Here's how the part is built. I have some questions about the finished solid (model axes, mm). A direction names the side the tool comes from. Coordinates: 2 decimals unless noted, no trailing zeros. Loops run counter-clockwise (first coordinate to the right, second up) from the corner with the lowest first, then second, coordinate; pieces in that order, holes last. Notation, with made-up numbers: (51.5, 4) - (76.5, 4) arc R13 ccw to (76.5, 20) - close; hole circle Ø8 at (-17, -17.75). An arc over 180 degrees is marked (long way). Use a Markdown table: item, result.
```python
from build123d import *
from build123d import SkipClean  # not in build123d's __all__

# Parameters (mm, degrees)
F0_R     = 10.7
F1_DEPTH = 30
F2_R     = 6
F4_DEPTH = 10.701
F5_DEPTH = 10.7010001
F6_W     = 6.2500013784
F6_H     = 36.9480545221
F6_W_2   = 6.8020046502
F6_H_2   = 40.0000055429
F7_DEPTH = 24
F8_R     = 2


# Not quite as in the source:
# - after a boolean that leaves OpenCascade's solid faulty, fix() repairs it


with BuildPart() as f1:
    # F0 (on Top) → F1 (new body)
    with BuildSketch(Plane.XY):
        Circle(F0_R)
    extrude(amount=-F1_DEPTH)

    # F2
    f2_edges = [f1.edges().sort_by_distance(p)[0] for p in [
        (-10.7, 0, -30),
    ]]
    fillet(f2_edges, radius=F2_R)

    # F3 (on Right) → F4 (cut, through all)
    with BuildSketch(Plane.YZ):
        with BuildLine():
            ThreePointArc((0, -12.2), (-3.3941125497, -20.3941125497), (4.8, -17))
            ThreePointArc((4.8, -17), (3.3941125497, -13.6058874503), (0, -12.2))
        make_face()
    extrude(amount=-F4_DEPTH, mode=Mode.SUBTRACT)

    # F5 (cut, through all): a face of the model
    f5_faces = [f1.faces().sort_by_distance(p)[0] for p in [
        (0, 0, -17),
    ]]
    with SkipClean():  # cleaning this boolean's faces spoils the solid; the shape is the same uncleaned
        extrude(f5_faces, amount=-F5_DEPTH, mode=Mode.SUBTRACT)

    # F6 (on face) → F7 (cut)
    with BuildSketch(Plane(origin=(0, 0, -30), x_dir=(1, 0, 0), z_dir=(0, 0, -1))):
        with Locations((-8.1250006892, 1.5259755104)):
            Rectangle(F6_W, F6_H)
        with Locations((8.4010023251, 0)):
            Rectangle(F6_W_2, F6_H_2)
    extrude(amount=-F7_DEPTH, mode=Mode.SUBTRACT)

    add(f1.part.fix(), mode=Mode.REPLACE)

    # F8
    f8_edges = [f1.edges().sort_by_distance(p)[0] for p in [
        (-5, 0, -6),
        (5, 0, -6),
    ]]
    fillet(f8_edges, radius=F8_R)


solid = f1.part
```
Q1. Please list where these lines run through material, in increasing order: L1, parallel to Z at x = 2.6, y = 0; L2, parallel to X at y = 0, z = -26.5; L3, parallel to Z at x = -1.25, y = 2.25. Write a range as from..to.
Check values:
| item | result |
|---|---|
| L1 | -30..-21.8, -12.2..0 |
| L2 | -5..5 |
| L3 | -30..-21.24, -12.76..0 |
Q2. I want a section at C-C, the plane z = -7. Write out the boundary of the cut face in (x, y), then the cut area to 3 significant figures.
Check values:
| item | result |
|---|---|
| outline | (-5.27, -9.31) arc R10.7 ccw to (5.27, -9.31) - (5.27, 9.31) arc R10.7 ccw to (-5.27, 9.31) - close |
| area | 216 mm^2 |
Q3. Which directions (+Z, -Z, +X, -X, +Y, -Y) give clear straight access to the entire face, cutting with the end or side of a thin tool? Please do faces 1 (the face through (0, 0, 0)), 2 (the face through (-8, 0, -6)), 3 (the face through (8, 0, -6)).
Check values:
| item | result |
|---|---|
| face 1 | +Z, +X, -X, +Y, -Y |
| face 2 | -Z, -X, +Y, -Y |
| face 3 | -Z, +X, +Y, -Y |
Q4. I want a section at A-A, the plane z = -21. Write out the boundary of the cut face in (x, y).
Check values:
| item | result |
|---|---|
| outline | (-5, -9.46) arc R10.7 ccw to (5, -9.46) - (5, -2.65) - (-5, -2.65) - close; (-5, 2.65) - (5, 2.65) - (5, 9.46) arc R10.7 ccw to (-5, 9.46) - close |
Q5. I want a section at B-B, the plane x = -6.25. Write out the boundary of the cut face in (y, z), then the cut area to 3 significant figures.
Check values:
| item | result |
|---|---|
| outline | (-8.68, -6.15) - (8.68, -6.15) - (8.68, 0) - (-8.68, 0) - close |
| area | 107 mm^2 |
Q6. Will these pins go through, and if not, where does the flat tip stop? P1, Ø3, axis at x = 9, y = -1.5, coming from the -Z side; P2, Ø4, axis at y = -7.5, z = -15.5, coming from the +X side; P3, Ø6, axis at x = 2, z = -20, coming from the -Y side; P4, Ø6, axis at y = 8.5, z = -25, coming from the -X side.
Check values:
| item | result |
|---|---|
| P1 | z = -6 |
| P2 | x = 5 |
| P3 | y = -10.7 |
| P4 | x = -5 |
